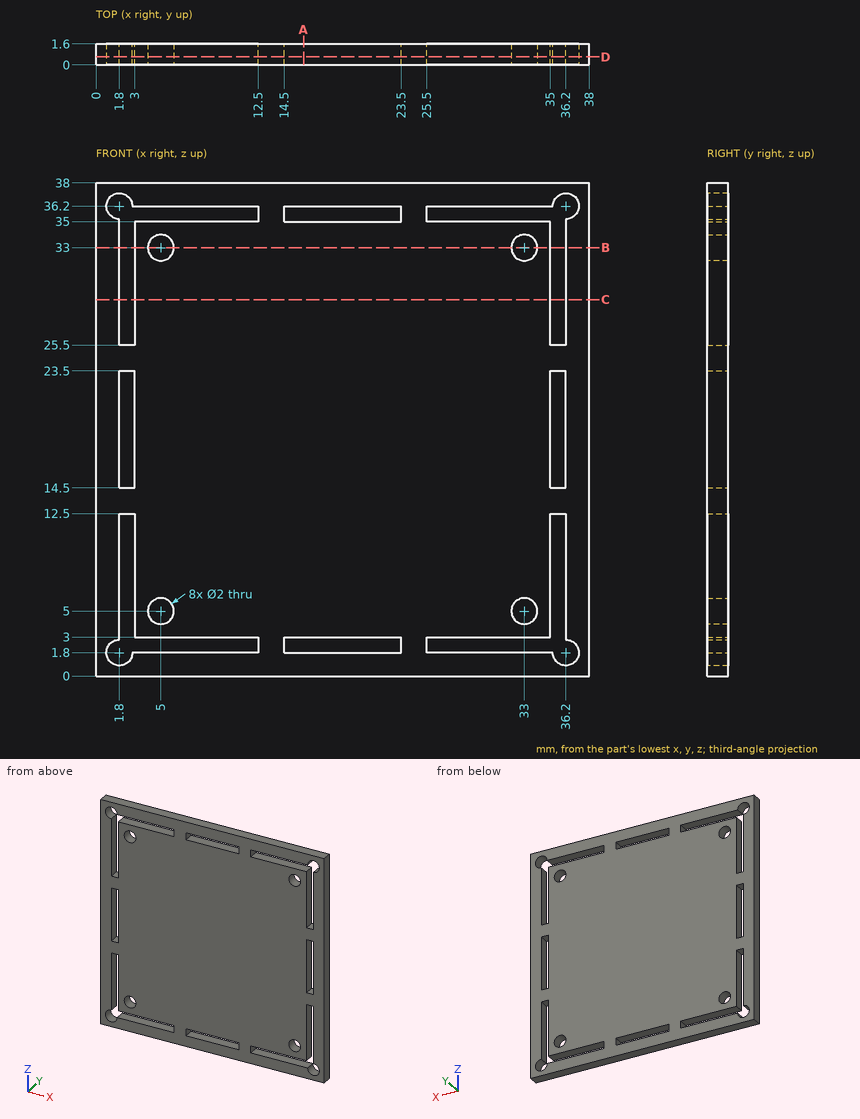
Input: dimensioned drawing with shaded views. Units: mm. Origin: part minimum x, y, z. Give positions to 0.01 mm unless a question says otherwise; leave off trailing zeros. Write each loop counter-clockwise with the first axis right and the second up, starting at its lowest first coordinate (ties: lowest second). Pieces come first, ordered by that corner, then holes. Notation, with made-up numbers: (-29, -20.5) - (5, -20.5) arc R23 cw to (5, 4.5) - close; hole circle Ø10 at (51, -5.75). An arc over 180 degrees is marked (long way). Write item = value, one per line. Start each with the question number.
1) Pin query (flat end, axial travel): pin 1 (1.8 mm diameter, centred on x = 5, z = 33, fed in from +Y); pin 2 (5 mm diameter, centred on x = 16, z = 29, fed in from -Y). Return the tip coordinate at first contact, or that it passes through.
2) Cut plane C-C (z = 29). Return loops of the section in (x, y), and give its area (3 significant figures).
3) Cut plane A-A (x = 16). Return loops of the section in (y, z), and give its area (3 significant figures).
4) Cut plane D-D (y = 0.6). Give the number of separate pieces and of enclosed holes in the cut face, and give its area (3 significant figures).
5) Cut plane B-B (z = 33). Return loops of the section in (x, y), and give its area (3 significant figures).
6) Material intervals for L1, parallel to Z at x = 5, y = 0.95; L2, parallel to X at y = 0.35, z = 21, sorted ascending. Write a range as [from, to].
Answers follow:
q1.pin_1 = through
q1.pin_2 = 0
q2.outline = (0, 0) - (1.8, 0) - (1.8, 1.6) - (0, 1.6) - close; (3, 0) - (35, 0) - (35, 1.6) - (3, 1.6) - close; (36.2, 0) - (38, 0) - (38, 1.6) - (36.2, 1.6) - close
q2.area = 57.0 mm^2
q3.outline = (0, 0) - (1.6, 0) - (1.6, 1.8) - (0, 1.8) - close; (0, 3) - (1.6, 3) - (1.6, 35) - (0, 35) - close; (0, 36.2) - (1.6, 36.2) - (1.6, 38) - (0, 38) - close
q3.area = 57.0 mm^2
q4.separate_pieces = 1
q4.enclosed_holes = 12
q4.area = 1,280 mm^2
q5.outline = (0, 0) - (1.8, 0) - (1.8, 1.6) - (0, 1.6) - close; (3, 0) - (4, 0) - (4, 1.6) - (3, 1.6) - close; (6, 0) - (32, 0) - (32, 1.6) - (6, 1.6) - close; (34, 0) - (35, 0) - (35, 1.6) - (34, 1.6) - close; (36.2, 0) - (38, 0) - (38, 1.6) - (36.2, 1.6) - close
q5.area = 50.6 mm^2
q6.L1 = [0, 1.8], [3, 4], [6, 32], [34, 35], [36.2, 38]
q6.L2 = [0, 1.8], [3, 35], [36.2, 38]
